Geometry check sheet. Reference: the model listing, model coordinates, mm. Face numbers are marked on the shaded views. A direction names the side the tool comes from. Give positions to 0.01 mm unless a question says otherwise; leave off trailing zeros. Write each loop counter-clockwise with the first axis right and the second up, starting at its lowest first coordinate (ties: lowest second). Pieces come first, ordered by that corner, then holes.
(1) Thickness scan on line 1 along Z through (x, y) = (-0.3, 0); line 2 along Y through (x, z) = (4.75, 11); line 3 along X through (y, z) = (0, 22). Record the ranges inside material, lowest first.
(2) Cross-section at A-A (y = 0). Record the boundary of the cut face in (x, z).
(3) Cross-section at B-B (x = 2.6). Record the boundary of the cut face in (y, z).
(4) Mould release check, pull along Y, two halves, no side actions. Record for the marked faces 1, 2 and 3: +Y half, -Y half, draft (parallel to the pull), parting line (faces both ways), or undercut.
(5) Depth check by flat-ended pin: P1, Ø5, axis at y = -0.5, z = 18, coming from the +X side; P2, Ø1.5, axis at x = 1.5, y = 1, coming from the +Z side; P3, Ø1.5, axis at x = 5, z = 19, coming from the +Y side; P4, Ø3, axis at y = 0, z = 15.04, coming from the -X side. Enter the tip coordinate at first touch or a pass-through.
(6) Tool access check on the marked faces 4, 5, 6, 7 and 8. Record the directions out of +Z, -Z, +X, -X, +Y, -Y that give a thin tool (end or side, any length) a straight path to the whole face; none if there is none.
(7) Cross-section at C-C (z = 28.5). Record the boundary of the cut face in (x, y).
(8) Cross-section at D-D (z = 3). Record the boundary of the cut face in (x, y) (3 decimals).
Autodesk Inventor part; units mm, degrees
ref_plane "YZ Plane" through (0, 0, 0) normal (1, 0, 0) x (0, 1, 0)
ref_plane "XZ Plane" through (0, 0, 0) normal (0, 1, 0) x (-1, 0, 0)
ref_plane "XY Plane" through (0, 0, 0) normal (0, 0, 1) x (1, 0, 0)
sketch "Sketch1" plane through (0, 0, 0) normal (1, 0, 0) x (0, 1, 0)
  line L0 (0, 0) -> (0, 15.0436) construction
  line L1 (-1.25, 0) -> (-1.25, 10)
  line L2 (1.25, 0) -> (1.25, 10)
  circle A0 centre (0, 15.0436) radius 2
  arc A1 (2.1667, 11.6812) -> (-2.1667, 11.6812) centre (0, 15.0436) ccw
  arc A2 (-1.25, 10) -> (-2.1667, 11.6812) centre (-3.25, 10) ccw
  arc A3 (2.1667, 11.6812) -> (1.25, 10) centre (3.25, 10) ccw
  line L3 (2.5, 20.0436) -> (-2.5, 20.0436) construction
  line L4 (-2.5, 20.0436) -> (-2.5, 30.0436) construction
  line L5 (-2.5, 30.0436) -> (2.5, 30.0436) construction
  line L6 (2.5, 30.0436) -> (2.5, 20.0436) construction
  line L7 (-6, 0) -> (6, 0)
  line L8 (6, 0) -> (6, 30.0436)
  line L9 (6, 30.0436) -> (-6, 30.0436)
  line L10 (-6, 30.0436) -> (-6, 0)
  line L11 (2.5, 0) -> (6, 13.0436)
  line L12 (6, 17.0436) -> (3.5, 30.0436)
  line L13 (6, 13.0436) -> (-6.1446, 13.0436) construction
  line L14 (6, 17.0436) -> (-6.1446, 17.0436) construction
  line L15 (-2.5, 0) -> (-6, 13.0436)
  line L16 (-6, 17.0436) -> (-3.5, 30.0436)
  point P0 (0, 20.0436)
  dimension "d0" = 2.5
  dimension "d1" = 4
  dimension "d2" = 2
  dimension "d3" = 2
  dimension "d4" = 10
  dimension "d5" = 10
  dimension "d6" = 5
  dimension "d7" = 1
  dimension "d8" = 2
  dimension "d9" = 2
  dimension "d10" = 7
extrude "Extrusion1" add sketch "Sketch1" along normal blind 7.2 contours L7 L15 L10 L16 L9 L12 L8 L11 L2 A3 A1 A2 L1
sketch "Sketch2" plane through (0, 0, 0) normal (-1, 0, 0) x (0, 0, 1)
  line L0 (0, -2.5) -> (0, -1.25)
  line L1 (0, 1.25) -> (0, 2.5)
  line L2 (0, 2.5) -> (13.0436, 6)
  line L3 (13.0436, 6) -> (17.0436, 6)
  line L4 (17.0436, 6) -> (30.0436, 3.5)
  line L5 (30.0436, 3.5) -> (30.0436, -3.5)
  line L6 (30.0436, -3.5) -> (17.0436, -6)
  line L7 (17.0436, -6) -> (13.0436, -6)
  line L8 (13.0436, -6) -> (0, -2.5)
  line L9 (0, -2.5) -> (0, -1.25)
  line L10 (0, 1.25) -> (0, -1.25)
  point P0 (0, 0)
extrude "Extrusion2" add sketch "Sketch2" along normal blind 2
sketch "Sketch3" plane through (-2, 0, 0) normal (-1, 0, 0) x (0, 0, 1)
  arc A0 (11.6812, -2.1667) -> (11.6812, 2.1667) centre (15.0436, 0) ccw
  point P0 (0, 0)
hole "Hole1" at (-2, 0, 15.0436) direction (1, 0, 0) diameter 3.4 end through all countersink diameter 6.3 countersink angle 90
sketch "Sketch4" plane through (7.2, -3.5, 30.0436) normal (0, 0, 1) x (1, 0, 0)
  line L0 (-9.2, 0) -> (0, 0) construction
  line L1 (0, 7) -> (0, 0) construction
  line L2 (-9.2, 7) -> (0, 7) construction
  line L3 (-9.2, 0) -> (-9.2, 7) construction
  line L4 (0, 7) -> (-9.2, 0) construction
  line L5 (-9.2, 7) -> (0, 0) construction
  point P0 (-7.2, 3.5)
  point P1 (-4.6, 3.5)
hole "Hole2" at (2.6, 0, 30.0436) direction (0, 0, -1) diameter 5 depth 10
equation "\"d9\" = d8"
properties part number "BeltClampM5"
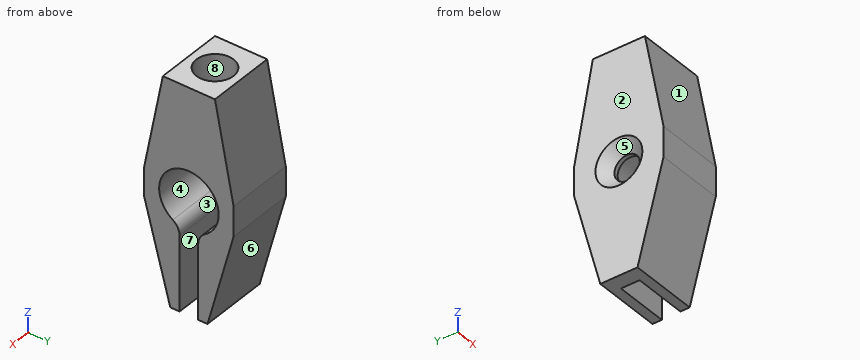
Reply:
1. line 1: z = 0 to 13.34, 16.74 to 30.04
1. line 2: y = -5.45 to -1.52, 1.52 to 5.45
1. line 3: x = -2 to 0.1, 5.1 to 7.2
2. outline: (-2, 0) - (0, 0) - (0, 13.34) - (-0.55, 13.34) - (-2, 11.89) - close; (-2, 18.19) - (-0.55, 16.74) - (0, 16.74) - (0, 19.04) - (7.2, 19.04) - (7.2, 30.04) - (5.1, 30.04) - (5.1, 20.04) - (0.1, 20.04) - (0.1, 30.04) - (-2, 30.04) - close
3. outline: (-6, 13.04) - (-2.5, 0) - (-1.25, 0) - (-1.25, 10) arc R2 ccw to (-2.17, 11.68) arc R4 cw (long way) to (2.17, 11.68) arc R2 ccw to (1.25, 10) - (1.25, 0) - (2.5, 0) - (6, 13.04) - (6, 17.04) - (3.5, 30.04) - (2.5, 30.04) - (2.5, 20.04) - (-2.5, 20.04) - (-2.5, 30.04) - (-3.5, 30.04) - (-6, 17.04) - close
4. face 1: -Y half
4. face 2: draft
4. face 3: undercut
5. P1: stops at x = 7.2
5. P2: stops at z = 20.04
5. P3: stops at y = 5.77
5. P4: passes through
6. face 4: +X
6. face 5: -X
6. face 6: -Z, +X, -X, +Y
6. face 7: -Z, +X
6. face 8: +Z
7. outline: (-2, -3.8) - (7.2, -3.8) - (7.2, 3.8) - (-2, 3.8) - close; hole circle Ø5 at (2.6, 0)
8. outline: (-2, -3.305) - (7.2, -3.305) - (7.2, -1.25) - (0, -1.25) - (0, 1.25) - (7.2, 1.25) - (7.2, 3.305) - (-2, 3.305) - close
